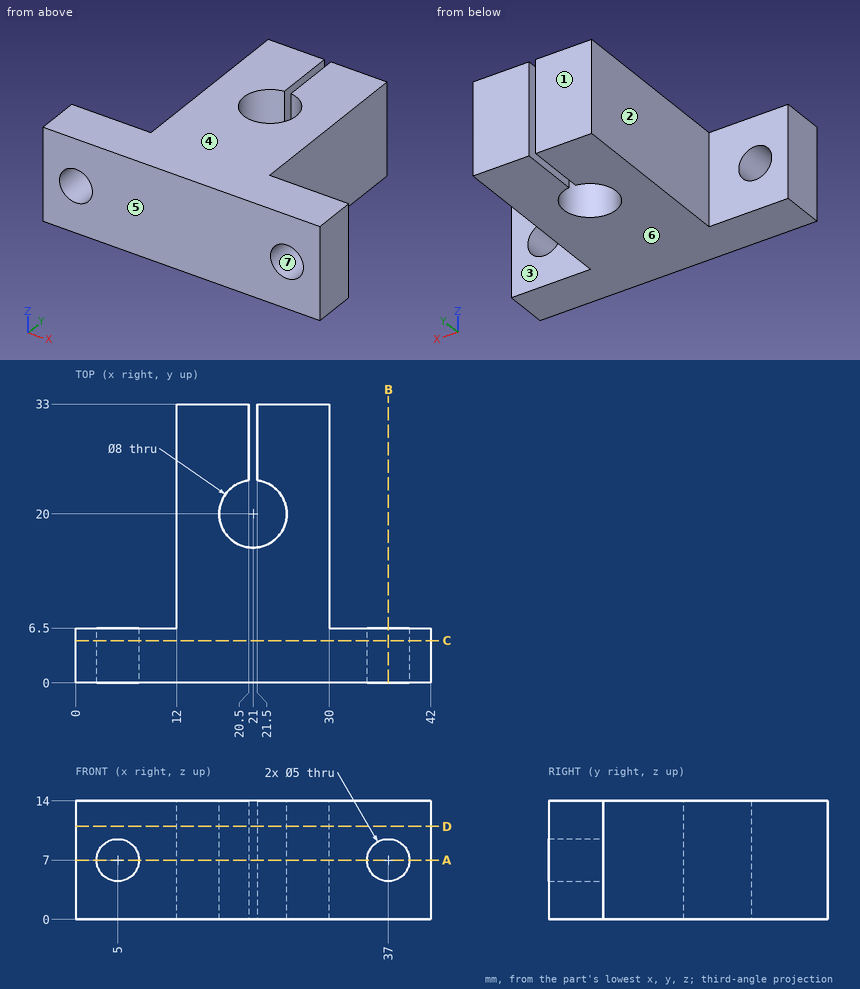
Drawing for the job (mm, zero at the part's lowest x, y, z). A direction names the side the tool comes from. Round coordinates to 2 decimals unless told otherwise and drop trailing zeros. Write each loop counter-clockwise with the first axis right and the second up, starting at its lowest first coordinate (ties: lowest second). Pieces come first, ordered by that corner, then holes. Notation, with made-up numbers: M 75,79 L 98,79 A25 cw 98,92 Z; hole C 26,27.25 d1. An arc over 180 degrees is marked long. Put each result on its own line as item: value.
Item 1: Cut at D-D (z = 11). List the corners of the cut face in (x, y).
Responses:
outline: M 0,0 L 42,0 L 42,6.5 L 30,6.5 L 30,33 L 21.5,33 L 21.5,23.97 A4 cw long 20.5,23.97 L 20.5,33 L 12,33 L 12,6.5 L 0,6.5 Z
Item 2: Mould opens along Z. For the marked faces 4, 5, 6 and 7 say: +Z half, -Z half, draft (parallel to the pull), parting line (faces both ways), or undercut.
Responses:
face 4: +Z half
face 5: draft
face 6: -Z half
face 7: undercut
Item 3: Cut at A-A (z = 7). List the corners of the cut face in (x, y).
Responses:
outline: M 0,0 L 2.5,0 L 2.5,6.5 L 0,6.5 Z; M 7.5,0 L 34.5,0 L 34.5,6.5 L 30,6.5 L 30,33 L 21.5,33 L 21.5,23.97 A4 cw long 20.5,23.97 L 20.5,33 L 12,33 L 12,6.5 L 7.5,6.5 Z; M 39.5,0 L 42,0 L 42,6.5 L 39.5,6.5 Z
Item 4: Probe L1, parallel to X at y = 2.75, z = 7; L2, parallel to X at y = 20, z = 3; L3, parallel to Z at x = 5, y = 4. List the from-to ranges inside material, lowest first. Write a range as from..to.
Responses:
L1: 0..2.5, 7.5..34.5, 39.5..42
L2: 12..17, 25..30
L3: 0..4.5, 9.5..14
Item 5: Cut at C-C (y = 5). List the corners of the cut face in (x, z), and give its area (3 significant figures).
Responses:
outline: M 0,0 L 42,0 L 42,14 L 0,14 Z; hole C 5,7 d5; hole C 37,7 d5
area: 549 mm²
Item 6: Flat gauge pins, fed straight in: P1, Ø5, axis at y = 21, z = 12, coming from the -X side; P2, Ø3.5, axis at x = 5.5, z = 7.5, coming from the +Y side; P3, Ø8, axis at x = 5, z = 7, coming from the +Y side; P4, Ø6, axis at y = 28, z = 10.5, coming from the +X side. Where does each tip first touch, or does it go through?
Responses:
P1: x = 12
P2: through
P3: y = 6.5
P4: x = 30
Item 7: Cut at B-B (x = 37). List the corners of the cut face in (y, z), and give its area (3 significant figures).
Responses:
outline: M 0,0 L 6.5,0 L 6.5,4.5 L 0,4.5 Z; M 0,9.5 L 6.5,9.5 L 6.5,14 L 0,14 Z
area: 58.5 mm²
Item 8: Tool access for the marked faces 1, 2 and 3: list every direction of +Z, -Z, +X, -X, +Y, -Y with a clear straight run to the whole face (end or side of a thin tool).
Responses:
face 1: +Z, -Z, +X, -X, +Y
face 2: +Z, -Z, -X, +Y
face 3: +Z, -Z, +X, +Y
